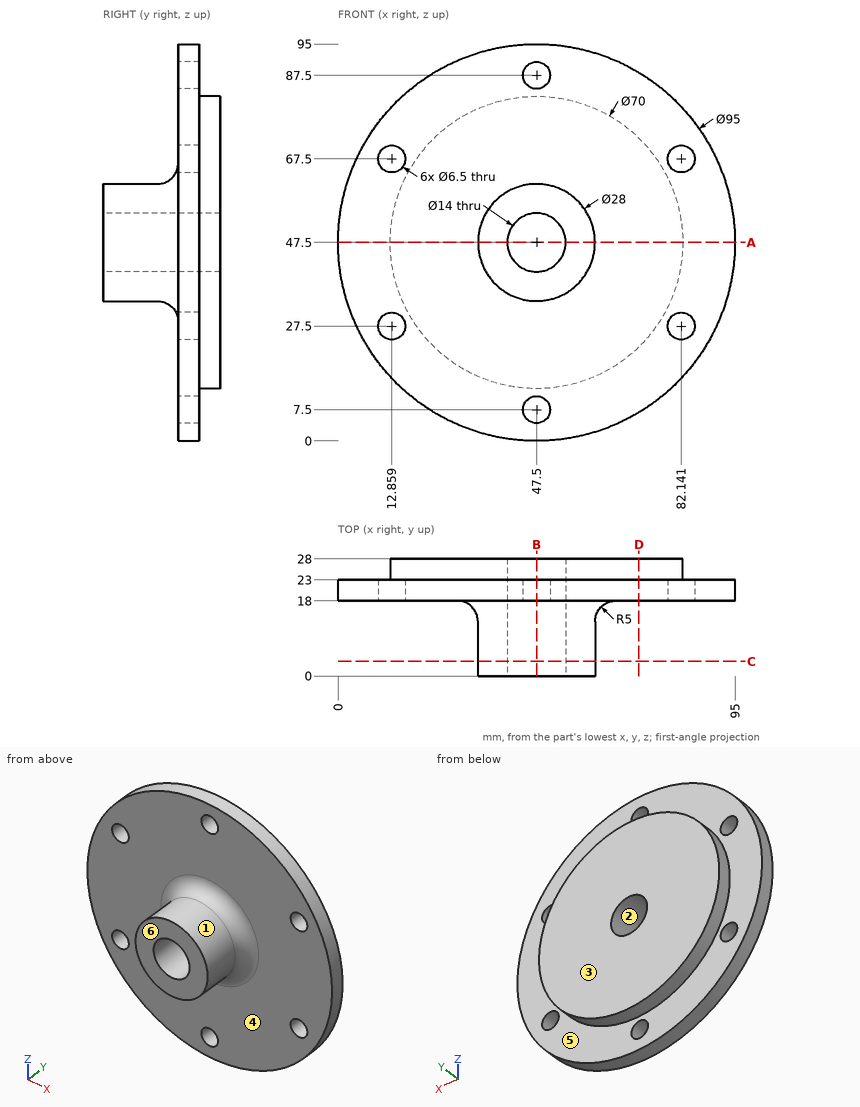
The drawing under review shows one solid part. Ordinate dimensions are in mm from its lowest x, y, z. A direction names the side the tool comes from. Round coordinates to 2 decimals unless told otherwise and drop trailing zeros. Loops run counter-clockwise (first coordinate to the right, second up) from the corner with the lowest first, then second, coordinate; pieces in that order, holes last. Notation, with made-up numbers: (62, 25.5) - (118, 25.5) arc R21 cw to (118, 30.5) - close; hole circle Ø7 at (43, 20.25). An arc over 180 degrees is marked (long way). One line per question, with ' | ' between items.
1. We need section D-D, the plane x = 72. State the section outline as (y, z) points (3 decimals).
Results are:
outline: (18, 6.806) - (23, 6.806) - (23, 22.505) - (28, 22.505) - (28, 72.495) - (23, 72.495) - (23, 88.194) - (18, 88.194) - close
2. For L1, parallel to Z at x = 47.5, y = 21.9; L2, parallel to X at y = 19.75, z = 27.5; L3, parallel to Y at x = 7, z = 71, list the stretches that pass through material, from the lowest coordinate up. Write a range as [from, to].
Results are:
L1: z = [0, 4.25], [10.75, 40.5], [54.5, 84.25], [90.75, 95] | L2: x = [4.42, 9.61], [16.11, 78.89], [85.39, 90.58] | L3: y = [18, 23]
3. We need section C-C, the plane y = 3.5. State the section outline as (x, z) points.
Results are:
outline: circle Ø28 at (47.5, 47.5); hole circle Ø14 at (47.5, 47.5)
4. We need section B-B, the plane x = 47.5. State the section outline as (y, z) points, and give its area (3 significant figures).
Results are:
outline: (0, 33.5) - (13, 33.5) arc R5 cw to (18, 28.5) - (18, 10.75) - (23, 10.75) - (23, 12.5) - (28, 12.5) - (28, 40.5) - (0, 40.5) - close; (0, 54.5) - (28, 54.5) - (28, 82.5) - (23, 82.5) - (23, 84.25) - (18, 84.25) - (18, 66.5) arc R5 cw to (13, 61.5) - (0, 61.5) - close; (18, 0) - (23, 0) - (23, 4.25) - (18, 4.25) - close; (18, 90.75) - (23, 90.75) - (23, 95) - (18, 95) - close | area: 883 mm²
5. For the marked faces 4, 5 and 6, list the 3-axis set-ups (+Z, -Z, +X, -X, +Y, -Y) from which the entire face can be reached by the end or side of a thin tool; tool diameter is ignored.
Results are:
face 4: -Y | face 5: +Y | face 6: +Z, -Z, +X, -X, -Y
6. Clearance check with flat-ended pins moving along their axes: P1, Ø7.5, axis at x = 12.86, z = 27.5, coming from the -Y side; P2, Ø10, axis at x = 82.5, z = 63, coming from the +Y side; P3, Ø6, axis at x = 47, y = 7.5, coming from the +Z side; P4, Ø1, axis at x = 17.5, y = 18, coming from the +Z side. State where each tip first meets the part, or that it passes through.
Results are:
P1: stops at y = 18 | P2: stops at y = 28 | P3: stops at z = 61.5 | P4: stops at z = 84.73
7. Draft analysis for pull direction X (two halves, no side actions). For the marked faces 1, 2 and 3, state which applies: released by +X, released by -X, zero draft, split by the parting line, or undercut.
Results are:
face 1: split by the parting line | face 2: undercut | face 3: zero draft
8. We need section A-A, the plane z = 47.5. State the section outline as (x, y) points.
Results are:
outline: (0, 18) - (28.5, 18) arc R5 cw to (33.5, 13) - (33.5, 0) - (40.5, 0) - (40.5, 28) - (12.5, 28) - (12.5, 23) - (0, 23) - close; (54.5, 0) - (61.5, 0) - (61.5, 13) arc R5 cw to (66.5, 18) - (95, 18) - (95, 23) - (82.5, 23) - (82.5, 28) - (54.5, 28) - close
